```python
from build123d import *
from build123d.topology import SkipClean

# Parameters (mm, degrees)
EXTRUDE_1_DEPTH     = 6
FILLET_3_RADIUS     = 3
FILLET_3_LENGTH     = 2
FILLET_4_RADIUS     = 3
FILLET_4_LENGTH     = 2.5
SKETCH_2_R          = 0.85
SKETCH_2_R_2        = 1.55
CUT_EXTRUDE_1_DEPTH = 40.357337308
EXTRUDE_START       = 3
SKETCH_3_R          = 3
SKETCH_3_R_2        = 1.55
EXTRUDE_2_DEPTH     = 3


with BuildPart() as part:
    # 草图1 → 凸台-拉伸1 (new body)
    with BuildSketch(Plane.XY):
        Polygon((-2, -2.5), (7.5, -2.5), (7.5, -37), (10, -37), (10, 0), (0, 0), (0, 20), (-2, 20), (-2, 8.273638366), align=None)
    extrude(amount=EXTRUDE_1_DEPTH)

    # 圆角3: full round fillet: the end face becomes a half cylinder, R = half its width
    fillet_3_face = Plane((-1, 20, 3), x_dir=(-1, 0, 0), z_dir=(0, 1, 0))  # on the end face: x along it, z out of the body
    fillet_3_slab = fillet_3_face.offset(-FILLET_3_RADIUS / 2) * Box(FILLET_3_LENGTH, 2 * FILLET_3_RADIUS, FILLET_3_RADIUS, mode=Mode.PRIVATE)  # the body's end, R deep
    fillet_3_round = Plane((-1, 17, 3), x_dir=(0, 1, 0), z_dir=(-1, 0, 0)) * Cylinder(FILLET_3_RADIUS, FILLET_3_LENGTH, mode=Mode.PRIVATE)  # its axis R under the face
    add(fillet_3_slab - fillet_3_round, mode=Mode.SUBTRACT)

    # 圆角4: full round fillet: the end face becomes a half cylinder, R = half its width
    fillet_4_face = Plane((8.75, -37, 3), x_dir=(-1, 0, 0), z_dir=(0, -1, 0))  # on the end face: x along it, z out of the body
    fillet_4_slab = fillet_4_face.offset(-FILLET_4_RADIUS / 2) * Box(FILLET_4_LENGTH, 2 * FILLET_4_RADIUS, FILLET_4_RADIUS, mode=Mode.PRIVATE)  # the body's end, R deep
    fillet_4_round = Plane((8.75, -34, 3), x_dir=(0, -1, 0), z_dir=(-1, 0, 0)) * Cylinder(FILLET_4_RADIUS, FILLET_4_LENGTH, mode=Mode.PRIVATE)  # its axis R under the face
    add(fillet_4_slab - fillet_4_round, mode=Mode.SUBTRACT)

    # 草图2 → 切除-拉伸1 (cut, through all)
    with BuildSketch(Plane.ZY.offset(2)):
        with Locations(Location((3, 17, 0), (0, 0, 270))):
            Circle(SKETCH_2_R)
        with Locations(Location((3, -34, 0), (0, 0, 270))):
            Circle(SKETCH_2_R_2)
    extrude(amount=-CUT_EXTRUDE_1_DEPTH, mode=Mode.SUBTRACT)

    # 草图3 → 凸台-拉伸2 (add)
    with SkipClean():  # the faces are left unmerged after this step: merging them gives an invalid solid
        with BuildSketch(Plane.ZY.offset(-7.5).offset(EXTRUDE_START)):
            with Locations(Location((3, -34, 0), (0, 0, 180))):
                Circle(SKETCH_3_R)
            with Locations(Location((3, -34, 0), (0, 0, 270))):
                Circle(SKETCH_3_R_2, mode=Mode.SUBTRACT)
        extrude(amount=-EXTRUDE_2_DEPTH)


solid = part.part
```
The model under review builds one solid part; all positions refer to its coordinate system, in mm. A direction names the side the tool comes from. Coordinates: 2 decimals unless noted, no trailing zeros. Write each loop counter-clockwise with the first axis right and the second up, starting at its lowest first coordinate (ties: lowest second). Pieces come first, ordered by that corner, then holes. Notation, with made-up numbers: (-15, 62.5) - (19, 62.5) arc R18 cw to (19, 83.5) - close; hole circle Ø6 at (25.5, -30). An arc over 180 degrees is marked (long way). Answer in a Markdown table with one row per item. Add a question column.
Q1. To check wall thickness, follow line 1 along Z through (x, y) = (-1, 17); line 2 along Z through (x, y) = (5.35, -34); line 3 along Y through (x, z) = (8.5, 3.05). State the ranges of each line that lie inside material, in increasing order. Write a range as from..to.
Q2. Draft analysis for pull direction Y (two halves, no side actions). For faces 4 (the face through (-1, 20, 3)), 5 (the face through (0, 10, 3)), 6 (the face through (3, -2.5, 3)), 7 (the face through (7.5, -18, 3)), state which applies: +Y half, -Y half, draft (parallel to the pull), parting line (faces both ways), or undercut.
Q3. Consider section D-D on z = 0.95. Give the boundary of the cut face in (x, y), then the cut area to 3 significant figures.
Q4. Clearance check with flat-ended pins moving along their axes: pin 1 (1.8 mm diameter, centred on y = -13.5, z = 4.5, fed in from -X); pin 2 (3 mm diameter, centred on y = -33.5, z = 4.5, fed in from -X); pin 3 (1.5 mm diameter, centred on y = 8, z = 5, fed in from +X). State where each tip first meets the part, or that it passes through.
Q5. Consider section A-A on x = 6.25. Give the boundary of the cut face in (y, z).
Q6. For faces 1 (the face through (5, 0, 3)), 2 (the face through (4.5, -32.7, 1.7)), 3 (the face through (10, -19, 3)), list the 3-axis set-ups (+Z, -Z, +X, -X, +Y, -Y) from which the entire face can be reached by the end or side of a thin tool; tool diameter is ignored.
Q7. Consider section B-B on z = 3. Give the boundary of the cut face in (x, y), then the cut area to 3 significant figures.
Q8. Consider section C-C on y = 5. Give the boundary of the cut face in (x, z), then the cut area to 3 significant figures.
Answers below:
| question | item | result |
|---|---|---|
| 1 | line 1 | 0..2.15, 3.85..6 |
| 1 | line 2 | 0..1.45, 4.55..6 |
| 1 | line 3 | -37..-35.55, -32.45..0 |
| 2 | face 4 | +Y half |
| 2 | face 5 | draft |
| 2 | face 6 | undercut |
| 2 | face 7 | undercut |
| 3 | outline | (-2, -2.5) - (7.5, -2.5) - (7.5, -31.81) - (4.5, -31.81) - (4.5, -36.19) - (10, -36.19) - (10, 0) - (0, 0) - (0, 19.19) - (-2, 19.19) - close |
| 3 | area | 166 mm² |
| 4 | pin 1 | x = 7.5 |
| 4 | pin 2 | x = 4.5 |
| 4 | pin 3 | x = 0 |
| 5 | outline | circle Ø6 at (-34, 3); (-2.5, 0) - (0, 0) - (0, 6) - (-2.5, 6) - close; hole circle Ø3.1 at (-34, 3) |
| 6 | face 1 | +Z, -Z, +X, +Y |
| 6 | face 2 | +Z, -Z, -X, -Y |
| 6 | face 3 | +Z, -Z, +X, +Y, -Y |
| 7 | outline | (-2, -2.5) - (7.5, -2.5) - (7.5, -31) - (4.5, -31) - (4.5, -32.45) - (10, -32.45) - (10, 0) - (0, 0) - (0, 16.15) - (-2, 16.15) - close; (-2, 17.85) - (0, 17.85) - (0, 20) - (-2, 20) - close; (4.5, -37) - (10, -37) - (10, -35.55) - (4.5, -35.55) - close |
| 7 | area | 154 mm² |
| 8 | outline | (-2, 0) - (0, 0) - (0, 6) - (-2, 6) - close |
| 8 | area | 12.0 mm² |
